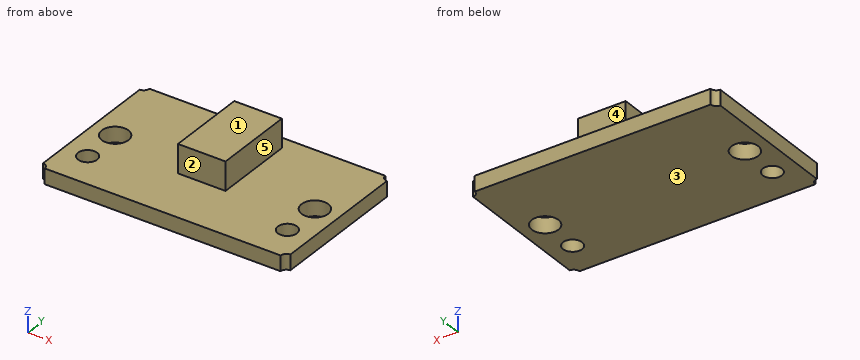
```python
from build123d import *

# Parameters (mm, degrees)
SKETCH1_W           = 26
SKETCH1_H           = 15.8
BOSS_EXTRUDE1_DEPTH = 1.61
SKETCH2_R           = 0.6
CUT_EXTRUDE1_DEPTH  = 1.61
SKETCH3_R           = 1.4
SKETCH3_R_2         = 1
CUT_EXTRUDE2_DEPTH  = 11.61
SKETCH4_W           = 5
SKETCH4_H           = 8.5
BOSS_EXTRUDE2_DEPTH = 3


with BuildPart() as part:
    # Sketch1 → Boss-Extrude1 (new body)
    with BuildSketch(Plane.XY):
        Rectangle(SKETCH1_W, SKETCH1_H)
    extrude(amount=BOSS_EXTRUDE1_DEPTH)

    # Sketch2 → Cut-Extrude1 (cut)
    with BuildSketch(Plane.XY.offset(1.61)):
        with Locations((-13, 7.9)):
            Circle(SKETCH2_R)
        with Locations((-13, -7.9)):
            Circle(SKETCH2_R)
        with Locations((13, -7.9)):
            Circle(SKETCH2_R)
        with Locations((13, 7.9)):
            Circle(SKETCH2_R)
    extrude(amount=-CUT_EXTRUDE1_DEPTH, mode=Mode.SUBTRACT)

    # Sketch3 → Cut-Extrude2 (cut)
    with BuildSketch(Plane.XY.offset(1.61)):
        with Locations((-10.5, 0)):
            Circle(SKETCH3_R)
        with Locations((10.5, 0)):
            Circle(SKETCH3_R)
        with Locations((-10.5, -4.15)):
            Circle(SKETCH3_R_2)
        with Locations((10.5, -4.15)):
            Circle(SKETCH3_R_2)
    extrude(amount=-CUT_EXTRUDE2_DEPTH, mode=Mode.SUBTRACT)

    # Sketch4 → Boss-Extrude2 (add)
    with BuildSketch(Plane.XY.offset(1.61)):
        with Locations((0, 2.25)):
            Rectangle(SKETCH4_W, SKETCH4_H)
    extrude(amount=BOSS_EXTRUDE2_DEPTH)


solid = part.part
```
Can you work these out from the model? Positions are in its coordinate system, mm. Face numbers are marked on the shaded views. A direction names the side the tool comes from. Give positions to 0.01 mm unless a question says otherwise; leave off trailing zeros. Loops run counter-clockwise (first coordinate to the right, second up) from the corner with the lowest first, then second, coordinate; pieces in that order, holes last. Notation, with made-up numbers: M 78,68.25 L 119,68.25 A3 ccw 119,72.25 Z; hole C 81,-24.5 d3. An arc over 180 degrees is marked long. One line per question, with ' | ' between items. Start each with the question number.
Q1. If I drill on line 1 (Y direction, x = -10.5, z = 0.4); line 2 (Z direction, x = 5.75, y = 5.5); line 3 (X direction, y = 3.5, z = 3), over which ranges is the centre line in solid material (lowest first)? Write a range as from..to.
Q2. If we section it at A-A (y = 0): Please give me the cut outline in (x, z), plus the area to 3 significant figures.
Q3. For pin 1 Ø1.5 at (x, z) = (0.5, 3.5) entering from -Y; pin 2 Ø1.5 at (x, y) = (-7.5, -1.5) entering from +Z; pin 3 Ø1.5 at (y, z) = (2.5, 3.5) entering from +X, each with a flat end and sliding along its axis, tell me the tip position at first contact or that it passes through.
Q4. If we section it at B-B (x = 10.5): Please give me the cut outline in (y, z).
Q5. For the marked faces 1, 2, 3, 4 and 5, which set-ups out of +Z, -Z, +X, -X, +Y, -Y let a thin tool reach every point of the face, with its end or its side?
Q6. If we section it at C-C (y = 1.75): Please give me the cut outline in (x, z).
Q7. If we section it at D-D (y = -4.15): Please give me the cut outline in (x, z).
Computed:
1) line 1: y = -7.9..-5.15, -3.15..-1.4, 1.4..7.9 | line 2: z = 0..1.61 | line 3: x = -2.5..2.5
2) outline: M -13,0 L -11.9,0 L -11.9,1.61 L -13,1.61 Z; M -9.1,0 L 9.1,0 L 9.1,1.61 L 2.5,1.61 L 2.5,4.61 L -2.5,4.61 L -2.5,1.61 L -9.1,1.61 Z; M 11.9,0 L 13,0 L 13,1.61 L 11.9,1.61 Z | area: 47.8 mm²
3) pin 1: stops at y = -2 | pin 2: stops at z = 1.61 | pin 3: stops at x = 2.5
4) outline: M -7.9,0 L -5.15,0 L -5.15,1.61 L -7.9,1.61 Z; M -3.15,0 L -1.4,0 L -1.4,1.61 L -3.15,1.61 Z; M 1.4,0 L 7.9,0 L 7.9,1.61 L 1.4,1.61 Z
5) face 1: +Z, +X, -X, +Y, -Y | face 2: +Z, +X, -X, -Y | face 3: -Z, +X, -X, +Y, -Y | face 4: +Z, +X, -X, +Y | face 5: +Z, +X, +Y, -Y
6) outline: M -13,0 L 13,0 L 13,1.61 L 2.5,1.61 L 2.5,4.61 L -2.5,4.61 L -2.5,1.61 L -13,1.61 Z
7) outline: M -13,0 L -11.5,0 L -11.5,1.61 L -13,1.61 Z; M -9.5,0 L 9.5,0 L 9.5,1.61 L -9.5,1.61 Z; M 11.5,0 L 13,0 L 13,1.61 L 11.5,1.61 Z
